```python
from build123d import *

# Parameters (mm, degrees)
SKETCH1_W               = 127
SKETCH1_H               = 342.9
BOSS_EXTRUDE1_DEPTH     = 12.7
DRAFT1_ANGLE            = -45
CUT_EXTRUDE1_DEPTH      = 184.272045059
CUT_EXTRUDE1_DEPTH_BACK = 5.08


with BuildPart() as part:
    # Sketch1 → Boss-Extrude1 (new body)
    with BuildSketch(Plane(origin=(0, 0, 0), x_dir=(0, 0, -1), z_dir=(1, 0, 0))):
        Rectangle(SKETCH1_W, SKETCH1_H)
    extrude(amount=BOSS_EXTRUDE1_DEPTH)

    # Draft1
    draft1_faces = [part.faces().sort_by_distance(p)[0] for p in [
        (6.35, -171.45, 0),
        (6.35, 0, -63.5),
        (6.35, 0, 63.5),
        (6.35, 171.45, 0),
    ]]
    draft(draft1_faces, Plane(origin=(0, 0, 0), x_dir=(0, 0, -1), z_dir=(-1, 0, 0)), DRAFT1_ANGLE)

    # Sketch2 → Cut-Extrude1 (cut, two sides: drawn at the far end of the back side and taken through both)
    with BuildSketch(Plane(origin=(12.7, 0, 0), x_dir=(0, 0, -1), z_dir=(1, 0, 0)).offset(-CUT_EXTRUDE1_DEPTH_BACK)):
        with BuildLine():
            Line((-63.5, 19.431), (-30.988, 19.431))
            ThreePointArc((-30.988, 19.431), (-24.384, 12.827), (-30.988, 6.223))
            Line((-30.988, 6.223), (-30.988, -0.508))
            Line((-30.988, -0.508), (63.5, -0.508))
            Line((63.5, -0.508), (63.5, -23.876))
            Line((63.5, -23.876), (-63.5, -23.876))
            Line((-63.5, -23.876), (-63.5, 19.431))
        make_face()
    extrude(amount=CUT_EXTRUDE1_DEPTH + CUT_EXTRUDE1_DEPTH_BACK, mode=Mode.SUBTRACT)


solid = part.part
```
Work out the finished part from the listing and answer in its coordinate system (mm). A direction names the side the tool comes from. Round coordinates to 2 decimals unless told otherwise and drop trailing zeros. Loops run counter-clockwise (first coordinate to the right, second up) from the corner with the lowest first, then second, coordinate; pieces in that order, holes last. Notation, with made-up numbers: M 70,-28 L 88,-28 A9 ccw 88,-20 Z; hole C 3.5,-0.5 d10. An arc over 180 degrees is marked long. One line per question, with ' | ' between items.
Q1. Find section B-B, the plane z = 41. Give the vertices of the cut face in (x, y), then the cut area to 3 significant figures.
Conclusion:
outline: M 0,-171.45 L 12.7,-158.75 L 12.7,-23.88 L 7.62,-23.88 L 7.62,19.43 L 12.7,19.43 L 12.7,158.75 L 0,171.45 Z | area: 3,970 mm2
Q2. The mould has two halves that part along Y. Classify faces 3 (the flat face through (6.26, -165.19, 0.89)), 4 (the flat face through (7.62, -7, 12)), 5 (the flat face through (0, 2, 1)): +Y half, -Y half, draft (parallel to the pull), parting line (faces both ways), or undercut.
Conclusion:
face 3: -Y half | face 4: undercut | face 5: draft
Q3. Find section A-A, the plane x = 10.5. Give the vertices of the cut face in (y, z).
Conclusion:
outline: M -160.95,-53 L -23.88,-53 L -23.88,53 L -160.95,53 Z; M -0.51,-53 L 160.95,-53 L 160.95,53 L 19.43,53 L 19.43,30.99 A6.6 cw 6.22,30.99 L -0.51,30.99 Z
Q4. Consider line 1 along Y through (x, z) = (9, 6.5); line 2 along X through (y, z) = (-8.5, 46.5); line 3 along Y through (x, z) = (10.5, -29). Determine where each line is inside the solid, lowest interval first. Write a range as from..to.
Conclusion:
line 1: y = -162.45..-23.88, -0.51..162.45 | line 2: x = 0..7.62 | line 3: y = -160.95..-23.88, -0.51..160.95
Q5. Each of these flat-tipped pins is pushed along its axis until it touches: pin 1 Ø4 at (x, z) = (9, -0.5) entering from +Y; pin 2 Ø3 at (x, z) = (11, 22) entering from -Y; pin 3 Ø5 at (x, z) = (9.5, -6.5) entering from -Y. Where does it stop, or does it pass through?
Conclusion:
pin 1: stops at y = 164.45 | pin 2: stops at y = -161.95 | pin 3: stops at y = -164.45
Q6. Find section D-D, the plane y = -52. Give the vertices of the cut face in (x, z), then the cut area to 3 significant figures.
Conclusion:
outline: M 0,-63.5 L 12.7,-50.8 L 12.7,50.8 L 0,63.5 Z | area: 1,450 mm2
Q7. A tool of negligible diameter and unlimited length cuts with its end or side. For faces 1 (the cylindrical face through (10.124, 12.972, 24.386)), 2 (the flat face through (12.7, -90, 1)), from which of +Z, -Z, +X, -X, +Y, -Y can it reach the whole face along a straight path? Write none if from no direction.
Conclusion:
face 1: +Z, +X | face 2: +Z, -Z, +X, +Y, -Y
Q8. Find section C-C, the plane z = -41.5. Give the vertices of the cut face in (x, y), then the cut area to 3 significant figures.
Conclusion:
outline: M 0,-171.45 L 12.7,-158.75 L 12.7,-23.88 L 7.62,-23.88 L 7.62,-0.51 L 12.7,-0.51 L 12.7,158.75 L 0,171.45 Z | area: 4,070 mm2
